from build123d import *

# Parameters (mm, degrees)
ESQUISSE1_W             = 26
ESQUISSE1_H             = 20
BOSS_EXTRU_1_DEPTH      = 3
ESQUISSE2_R             = 1
ENL_V_MAT_EXTRU_1_DEPTH = 10
ESQUISSE3_W             = 9
ESQUISSE3_H             = 4
BOSS_EXTRU_2_DEPTH      = 20
ESQUISSE10_W            = 9
ESQUISSE10_H            = 10
BOSS_EXTRU_3_DEPTH      = 10
ENL_V_MAT_EXTRU_9_DEPTH = 5
ESQUISSE13_W            = 3
ESQUISSE13_H            = 20
BOSS_EXTRU_4_DEPTH      = 5


with BuildPart() as part:
    # Esquisse1 → Boss.-Extru.1 (new body)
    with BuildSketch(Plane.XY):
        with Locations((-10.76504298, -2.606017192)):
            Rectangle(ESQUISSE1_W, ESQUISSE1_H)
    extrude(amount=BOSS_EXTRU_1_DEPTH)

    # Esquisse2 → Enlèv. mat.-Extru.1 (cut)
    with BuildSketch(Plane.XY.offset(3)):
        with Locations((-20.77504298, -2.606017192)):
            Circle(ESQUISSE2_R)
        with Locations((1.22495702, -2.606017192)):
            Circle(ESQUISSE2_R)
    extrude(amount=-ENL_V_MAT_EXTRU_1_DEPTH, mode=Mode.SUBTRACT)

    # Esquisse3 → Boss.-Extru.2 (add)
    with BuildSketch(Plane.XY.offset(3)):
        with Locations((-5.76504298, -2.606017192)):
            Rectangle(ESQUISSE3_W, ESQUISSE3_H)
    extrude(amount=BOSS_EXTRU_2_DEPTH)

    # Esquisse10 → Boss.-Extru.3 (add)
    with BuildSketch(Plane(origin=(0, -4.606017192, 0), x_dir=(-1, 0, 0), z_dir=(0, -1, 0))):
        with Locations((5.76504298, -18)):
            Rectangle(ESQUISSE10_W, ESQUISSE10_H)
    extrude(amount=BOSS_EXTRU_3_DEPTH)

    # Esquisse12 → Enlèv. mat.-Extru.9 (cut)
    with BuildSketch(Plane.XZ.offset(14.606017192)):
        with BuildLine():
            Line((-1.76504298, 18), (-2.862370428, 18.757952542))
            ThreePointArc((-2.862370428, 18.757952542), (-2.867078041, 18.775757187), (-2.871894865, 18.793532598))
            Line((-2.871894865, 18.793532598), (-2.300941365, 20))
            Line((-2.300941365, 20), (-3.630231082, 20.107742433))
            ThreePointArc((-3.630231082, 20.107742433), (-3.643210317, 20.120807901), (-3.656269514, 20.133793446))
            Line((-3.656269514, 20.133793446), (-3.76504298, 21.464101615))
            Line((-3.76504298, 21.464101615), (-4.970112861, 20.89276444))
            ThreePointArc((-4.970112861, 20.89276444), (-4.987885942, 20.89758985), (-5.005688311, 20.902306063))
            Line((-5.005688311, 20.902306063), (-5.76504298, 22))
            Line((-5.76504298, 22), (-6.522995522, 20.902672552))
            ThreePointArc((-6.522995522, 20.902672552), (-6.540800167, 20.897964939), (-6.558575577, 20.893148115))
            Line((-6.558575577, 20.893148115), (-7.76504298, 21.464101615))
            Line((-7.76504298, 21.464101615), (-7.872785412, 20.134811898))
            ThreePointArc((-7.872785412, 20.134811898), (-7.885850881, 20.121832663), (-7.898836426, 20.108773466))
            Line((-7.898836426, 20.108773466), (-9.229144595, 20))
            Line((-9.229144595, 20), (-8.65780742, 18.794930119))
            ThreePointArc((-8.65780742, 18.794930119), (-8.66263283, 18.777157038), (-8.667349043, 18.759354669))
            Line((-8.667349043, 18.759354669), (-9.76504298, 18))
            Line((-9.76504298, 18), (-8.667715532, 17.242047458))
            ThreePointArc((-8.667715532, 17.242047458), (-8.663007919, 17.224242813), (-8.658191095, 17.206467402))
            Line((-8.658191095, 17.206467402), (-9.229144595, 16))
            Line((-9.229144595, 16), (-7.899854878, 15.892257567))
            ThreePointArc((-7.899854878, 15.892257567), (-7.886875643, 15.879192099), (-7.873816446, 15.866206554))
            Line((-7.873816446, 15.866206554), (-7.76504298, 14.535898385))
            Line((-7.76504298, 14.535898385), (-6.559973099, 15.10723556))
            ThreePointArc((-6.559973099, 15.10723556), (-6.542200018, 15.10241015), (-6.524397649, 15.097693937))
            Line((-6.524397649, 15.097693937), (-5.76504298, 14))
            Line((-5.76504298, 14), (-5.007090438, 15.097327448))
            ThreePointArc((-5.007090438, 15.097327448), (-4.989285793, 15.102035061), (-4.971510382, 15.106851885))
            Line((-4.971510382, 15.106851885), (-3.76504298, 14.535898385))
            Line((-3.76504298, 14.535898385), (-3.657300547, 15.865188102))
            ThreePointArc((-3.657300547, 15.865188102), (-3.644235079, 15.878167337), (-3.631249534, 15.891226534))
            Line((-3.631249534, 15.891226534), (-2.300941365, 16))
            Line((-2.300941365, 16), (-2.87227854, 17.205069881))
            ThreePointArc((-2.87227854, 17.205069881), (-2.86745313, 17.222842962), (-2.862736916, 17.240645331))
            Line((-2.862736916, 17.240645331), (-1.76504298, 18))
        make_face()
    extrude(amount=-ENL_V_MAT_EXTRU_9_DEPTH, mode=Mode.SUBTRACT)

    # Esquisse13 → Boss.-Extru.4 (add)
    with BuildSketch(Plane(origin=(2.23495702, 0, 0), x_dir=(0, 0, -1), z_dir=(1, 0, 0))):
        with Locations((-1.5, -2.606017192)):
            Rectangle(ESQUISSE13_W, ESQUISSE13_H)
    extrude(amount=BOSS_EXTRU_4_DEPTH)


solid = part.part
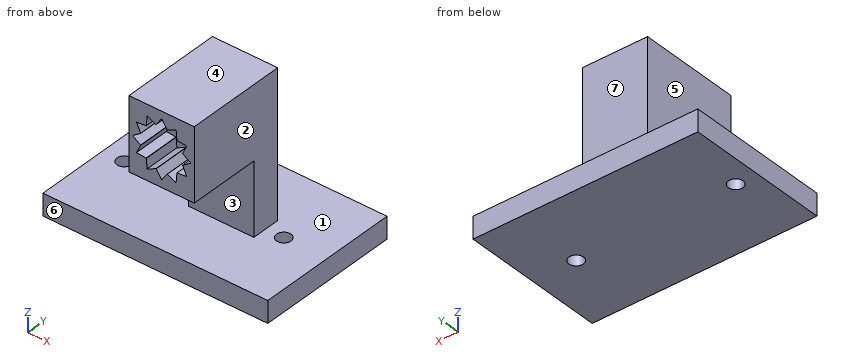
For this review, take the finished solid that the model builds, in its own axes (mm). Face numbers are marked on the shaded views. A direction names the side the tool comes from. Round coordinates to 2 decimals unless told otherwise and drop trailing zeros. Loops run counter-clockwise (first coordinate to the right, second up) from the corner with the lowest first, then second, coordinate; pieces in that order, holes last. Notation, with made-up numbers: (5.25, -30) - (63.25, -30) arc R26 ccw to (63.25, 9) - close; hole circle Ø1 at (-11, 62.5). An arc over 180 degrees is marked (long way). Use one line per item in the form item = value.
1) We need section B-B on x = 1.5. Write out the cut boundary in (y, z).
Solutions:
outline = (-12.61, 0) - (-3.57, 0) - (-3.57, 3) - (-12.61, 3) - close; (-1.64, 0) - (7.39, 0) - (7.39, 3) - (-1.64, 3) - close
2) We need section A-A on y = -7.5. Write out the cut boundary in (x, z).
Solutions:
outline = (-23.77, 0) - (7.23, 0) - (7.23, 3) - (-23.77, 3) - close; (-10.27, 13) - (-1.27, 13) - (-1.27, 23) - (-10.27, 23) - close
3) Wall thickness on probe 1 along Z at (x, y) = (-5.5, -8.5); probe 2 along Z at (x, y) = (-23, 6); probe 3 along Y at (x, z) = (-9, 19.25): over which ranges is each line inside the solid? List them lowest first.
Solutions:
probe_1 = 0 to 3, 13 to 23
probe_2 = 0 to 3
probe_3 = -14.61 to -0.61
4) We need section C-C on y = -12.25. State how many separate pieces and enclosed holes the cut face has, then the cut area to 3 significant figures.
Solutions:
separate_pieces = 2
enclosed_holes = 1
area = 146 mm2
5) We need section D-D on z = 20.5. Write out the cut boundary in (x, y), then the cut area to 3 significant figures.
Solutions:
outline = (-10.27, -14.61) - (-7.84, -14.61) - (-7.84, -9.61) - (-3.69, -9.61) - (-3.69, -14.61) - (-1.27, -14.61) - (-1.27, -0.61) - (-10.27, -0.61) - close
area = 105 mm2
6) Clearance check with flat-ended pins moving along their axes: P1, Ø2.5, axis at x = -20.78, y = -2.61, coming from the +Z side; P2, Ø3, axis at x = -10, z = 14.5, coming from the +Y side; P3, Ø4, axis at y = -7, z = 15.5, coming from the +X side. State where each tip first meets the part, or that it passes through.
Solutions:
P1 = 3
P2 = -0.61
P3 = -1.27
7) Mouldability with a two-part tool opening along Z and no side actions: class the marked faces 1, 2, 3 and 4 as pulls with the +Z half, pulls with the -Z half, needs draft (parallel to the pull), parting line crosses it, or undercut.
Solutions:
face_1 = undercut
face_2 = needs draft
face_3 = undercut
face_4 = pulls with the +Z half
8) Tool access review of the marked faces 5, 6 and 7: name each direction out of +Z, -Z, +X, -X, +Y, -Y from which nothing blocks a thin tool from reaching the whole face with its end or side.
Solutions:
face_5 = +Z, -X, +Y, -Y
face_6 = -Z, +X, -X, -Y
face_7 = +Z, +X, -X, +Y
